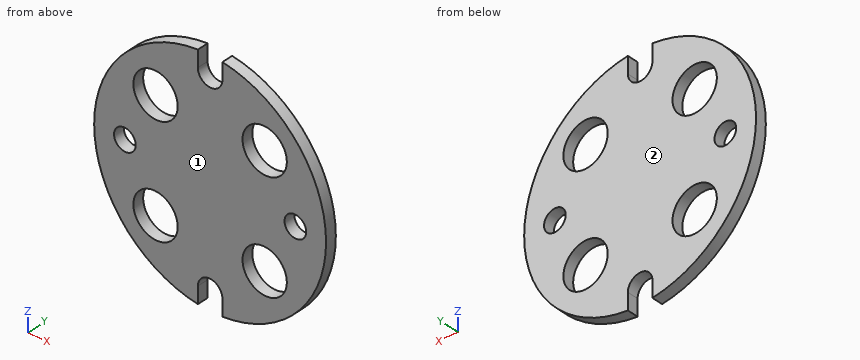
```python
from build123d import *

# Parameters (mm, degrees)
SKETCH1_R           = 17
BOSS_EXTRUDE1_DEPTH = 1.6
SKETCH2_R           = 1.59
SKETCH2_R_2         = 3.25
CUT_EXTRUDE1_DEPTH  = 25.09481272


with BuildPart() as part:
    # Sketch1 → Boss-Extrude1 (new body)
    with BuildSketch(Plane(origin=(0, 0, 0), x_dir=(1, 0, 0), z_dir=(0, 1, 0))):
        with Locations(Location((0, 0, 0), (0, 0, 270))):
            Circle(SKETCH1_R)
    extrude(amount=BOSS_EXTRUDE1_DEPTH)

    # Sketch2 → Cut-Extrude1 (cut, through all)
    with BuildSketch(Plane.XZ):
        with Locations(Location((12.5, 0, 0), (0, 0, 270))):
            Circle(SKETCH2_R)
        with Locations(Location((-12.5, 0, 0), (0, 0, 270))):
            Circle(SKETCH2_R)
        with Locations(Location((8, 8, 0), (0, 0, 270))):
            Circle(SKETCH2_R_2)
        with Locations(Location((8, -8, 0), (0, 0, 270))):
            Circle(SKETCH2_R_2)
        with Locations(Location((-8, -8, 0), (0, 0, 270))):
            Circle(SKETCH2_R_2)
        with Locations(Location((-8, 8, 0), (0, 0, 270))):
            Circle(SKETCH2_R_2)
        with BuildLine():
            Line((-1.8, 14.5), (-1.8, 16.904437287))
            ThreePointArc((-1.8, 16.904437287), (0, 17), (1.8, 16.904437287))
            Line((1.8, 16.904437287), (1.8, 14.5))
            ThreePointArc((1.8, 14.5), (0, 12.7), (-1.8, 14.5))
        make_face()
        with BuildLine():
            Line((1.8, -14.5), (1.8, -16.904437287))
            ThreePointArc((1.8, -16.904437287), (0, -17), (-1.8, -16.904437287))
            Line((-1.8, -16.904437287), (-1.8, -14.5))
            ThreePointArc((-1.8, -14.5), (0, -12.7), (1.8, -14.5))
        make_face()
    extrude(amount=-CUT_EXTRUDE1_DEPTH, mode=Mode.SUBTRACT)


solid = part.part
```
Geometry: final body of the model. Coordinates: model frame, mm. Face numbers are marked on the shaded views. Coordinates: 2 decimals unless noted, no trailing zeros. Order: outer loops, then holes, each group sorted by start corner. A loop starts at its lowest first (then second) coordinate and runs counter-clockwise, first axis right, second up.
Item 1: Section query A-A (x = 8). Output: boundary loops of the cut face in (y, z), then the cut area to 3 significant figures.
Answer:
outline: (0, -15) - (1.6, -15) - (1.6, -11.25) - (0, -11.25) - close; (0, -4.75) - (1.6, -4.75) - (1.6, 4.75) - (0, 4.75) - close; (0, 11.25) - (1.6, 11.25) - (1.6, 15) - (0, 15) - close
area: 27.2 mm2
Item 2: Draft query along Y for the marked faces 1 and 2. Return one class per face: released by +Y, released by -Y, zero draft, split by the parting line, or undercut.
Answer:
face 1: released by -Y
face 2: released by +Y
Item 3: Contact query for flat-ended pins moving along their axis: P1, Ø6, axis at x = -8.5, z = -6, coming from the -Y side; P2, Ø0.5, axis at y = 0.5, z = 15.5, coming from the +X side. Output: stop coordinate, or through.
Answer:
P1: stops at y = 0
P2: stops at x = 7.51
Item 4: Section query D-D (x = -12.5). Output: boundary loops of the cut face in (y, z), then the cut area to 3 significant figures.
Answer:
outline: (0, -11.52) - (1.6, -11.52) - (1.6, -1.59) - (0, -1.59) - close; (0, 1.59) - (1.6, 1.59) - (1.6, 11.52) - (0, 11.52) - close
area: 31.8 mm2
Item 5: Section query B-B (z = -8). Output: boundary loops of the cut face in (x, y), then the cut area to 3 significant figures.
Answer:
outline: (-15, 0) - (-11.25, 0) - (-11.25, 1.6) - (-15, 1.6) - close; (-4.75, 0) - (4.75, 0) - (4.75, 1.6) - (-4.75, 1.6) - close; (11.25, 0) - (15, 0) - (15, 1.6) - (11.25, 1.6) - close
area: 27.2 mm2
Item 6: Section query C-C (y = 1.05). Output: boundary loops of the cut face in (x, z).
Answer:
outline: (-1.8, -16.9) - (-1.8, -14.5) arc R1.8 cw to (1.8, -14.5) - (1.8, -16.9) arc R17 ccw to (1.8, 16.9) - (1.8, 14.5) arc R1.8 cw to (-1.8, 14.5) - (-1.8, 16.9) arc R17 ccw to start; hole circle Ø3.18 at (-12.5, 0); hole circle Ø6.5 at (-8, -8); hole circle Ø6.5 at (-8, 8); hole circle Ø6.5 at (8, -8); hole circle Ø6.5 at (8, 8); hole circle Ø3.18 at (12.5, 0)
Item 7: Material intervals for line 1 along X through (y, z) = (0.9, 0); line 2 along Z through (x, y) = (-9.5, 0.6); line 3 along X through (y, z) = (0.65, -0.5), sorted ascending.
Answer:
line 1: x = -17 to -14.09, -10.91 to 10.91, 14.09 to 17
line 2: z = -14.1 to -10.88, -5.12 to 5.12, 10.88 to 14.1
line 3: x = -16.99 to -14.01, -10.99 to 10.99, 14.01 to 16.99
